```python
from build123d import *

# Parameters (mm, degrees)
SKETCH_1_R          = 25
SKETCH_1_R_2        = 1.525
SKETCH_1_R_3        = 15
EXTRUDE_1_DEPTH     = 3
EXTRUDE_START       = -3
EXTRUDE_2_DEPTH     = 3
FILLET_1_R          = 3
SKETCH_4_R          = 1.515
CUT_EXTRUDE_1_DEPTH = 10


with BuildPart() as part:
    # 草图1 → 凸台-拉伸1 (new body)
    with BuildSketch(Plane.XY):
        Circle(SKETCH_1_R)
        with Locations((0, 20)):
            Circle(SKETCH_1_R_2, mode=Mode.SUBTRACT)
        with Locations((17.320508076, 10)):
            Circle(SKETCH_1_R_2, mode=Mode.SUBTRACT)
        with Locations((17.320508076, -10)):
            Circle(SKETCH_1_R_2, mode=Mode.SUBTRACT)
        with Locations((0, -20)):
            Circle(SKETCH_1_R_2, mode=Mode.SUBTRACT)
        with Locations((-17.320508076, -10)):
            Circle(SKETCH_1_R_2, mode=Mode.SUBTRACT)
        with Locations((-17.320508076, 10)):
            Circle(SKETCH_1_R_2, mode=Mode.SUBTRACT)
        Circle(SKETCH_1_R_3, mode=Mode.SUBTRACT)
    extrude(amount=EXTRUDE_1_DEPTH)

    # 草图3 → 凸台-拉伸2 (add)
    with BuildSketch(Plane.XY.offset(3).offset(EXTRUDE_START)):
        with BuildLine():
            Line((15, 20), (40, 20))
            Line((40, 20), (40, -20))
            Line((40, -20), (15, -20))
            ThreePointArc((15, -20), (25, 0), (15, 20))
        make_face()
        with BuildLine():
            Line((-40, -20), (-15, -20))
            ThreePointArc((-15, -20), (-25, 0), (-15, 20))
            Line((-15, 20), (-40, 20))
            Line((-40, 20), (-40, -20))
        make_face()
    extrude(amount=EXTRUDE_2_DEPTH)

    # 圆角1
    fillet_1_edges = [part.edges().sort_by_distance(p)[0] for p in [
        (40, 20, 1.5),
        (40, -20, 1.5),
        (15, -20, 1.5),
        (15, 20, 1.5),
        (-40, -20, 1.5),
        (-40, 20, 1.5),
        (-15, 20, 1.5),
        (-15, -20, 1.5),
    ]]
    fillet(fillet_1_edges, radius=FILLET_1_R)

    # 草图4 → 切除-拉伸1 (cut)
    with BuildSketch(Plane.XY.offset(3)):
        with Locations((-34, 15)):
            Circle(SKETCH_4_R)
        with Locations((-34, -5)):
            Circle(SKETCH_4_R)
        with Locations((34, -5)):
            Circle(SKETCH_4_R)
        with Locations((34, 15)):
            Circle(SKETCH_4_R)
    extrude(amount=-CUT_EXTRUDE_1_DEPTH, mode=Mode.SUBTRACT)


solid = part.part
```
Work out the finished part from the listing and answer in its coordinate system (mm). A direction names the side the tool comes from. Coordinates: 2 decimals unless noted, no trailing zeros. Write each loop counter-clockwise with the first axis right and the second up, starting at its lowest first coordinate (ties: lowest second). Pieces come first, ordered by that corner, then holes. Notation, with made-up numbers: (8, 76) - (39, 76) arc R24 cw to (39, 109) - close; hole circle Ø10 at (78.25, -36.5). An arc over 180 degrees is marked (long way). Answer as a JSON object with one key per item and string values.
Q1. For a pull along Y with two mould halves and no side action, classify faces 1 (the flat face through (40, 0, 1)), 2 (the cylindrical face through (0, -25, 1)), 3 (the cylindrical face through (-14.985, 0.66, 1.479)) as pulls with the +Y half, pulls with the -Y half, needs draft (parallel to the pull), parting line crosses it, or undercut.
Results list:
{"face 1": "needs draft", "face 2": "pulls with the -Y half", "face 3": "undercut"}
Q2. Find section A-A (x = 34). Write down the section's boundary in (y, z) (3 decimals), plus the area to 3 significant figures.
Results list:
{"outline": "(-20, 0) - (-6.515, 0) - (-6.515, 3) - (-20, 3) - close; (-3.485, 0) - (13.485, 0) - (13.485, 3) - (-3.485, 3) - close; (16.515, 0) - (20, 0) - (20, 3) - (16.515, 3) - close", "area": "102 mm^2"}
Q3. Find section C-C (y = 0). Write down the section's boundary in (x, z).
Results list:
{"outline": "(-40, 0) - (-15, 0) - (-15, 3) - (-40, 3) - close; (15, 0) - (40, 0) - (40, 3) - (15, 3) - close"}
Q4. Find section D-D (x = -10). Write down the section's boundary in (y, z), plus the area to 3 significant figures.
Results list:
{"outline": "(-22.91, 0) - (-11.18, 0) - (-11.18, 3) - (-22.91, 3) - close; (11.18, 0) - (22.91, 0) - (22.91, 3) - (11.18, 3) - close", "area": "70.4 mm^2"}
Q5. Consider L1, parallel to Y at x = 17.5, z = 2.1; L2, parallel to Y at x = -34, z = 1.15 (3 decimals); L3, parallel to X at y = -11, z = 2.85. Determine where each line is inside the solid, lowest interval first. Write a range as from..to.
Results list:
{"L1": "y = -20..-11.51, -8.49..8.49, 11.51..20", "L2": "y = -20..-6.515, -3.485..13.485, 16.515..20", "L3": "x = -40..-18.47, -16.17..-10.2, 10.2..16.17, 18.47..40"}
Q6. Given pin 1 Ø1.8 at (x, y) = (-17.32, 10) entering from +Z; pin 2 Ø0.9 at (x, z) = (27, 1) entering from -Y, each flat-ended and moving along its own axis, determine where each tip first touches the part or whether it passes through.
Results list:
{"pin 1": "passes through", "pin 2": "stops at y = -20"}
Q7. Find section B-B (z = 1.45). State how many separate pieces and enclosed holes the cut face has, plus the area to 3 significant figures.
Results list:
{"separate pieces": "1", "enclosed holes": "11", "area": "2,620 mm^2"}
Q8. Which of the six approach directions +Z, -Z, +X, -X, +Y, -Y give full straight-line access (tool end or side, diameter ignored) to faces 4 (the flat face through (27, -20, 1)), 5 (the flat face through (-27, -20, 1)), 6 (the flat face through (26, 20, 1))?
Results list:
{"face 4": "+Z, -Z, +X, -Y", "face 5": "+Z, -Z, -X, -Y", "face 6": "+Z, -Z, +X, +Y"}
